```python
from build123d import *

# Parameters (mm, degrees)
SKETCH_1_W          = 855
SKETCH_1_H          = 1200
SKETCH_1_W_2        = 695
SKETCH_1_H_2        = 1040
EXTRUDE_1_DEPTH     = 200
SKETCH_2_W          = 715
SKETCH_2_H          = 1060
CUT_EXTRUDE_1_DEPTH = 10


with BuildPart() as part:
    # Эскиз1 → Вытянуть-Тонкостенный1 (new body)
    with BuildSketch(Plane(origin=(0, 0, 0), x_dir=(1, 0, 0), z_dir=(0, 1, 0))):
        Rectangle(SKETCH_1_W, SKETCH_1_H)
        Rectangle(SKETCH_1_W_2, SKETCH_1_H_2, mode=Mode.SUBTRACT)
    extrude(amount=EXTRUDE_1_DEPTH)

    # Эскиз2 → Вырез-Вытянуть1 (cut)
    with BuildSketch(Plane(origin=(0, 200, 0), x_dir=(1, 0, 0), z_dir=(0, 1, 0))):
        Rectangle(SKETCH_2_W, SKETCH_2_H)
    extrude(amount=-CUT_EXTRUDE_1_DEPTH, mode=Mode.SUBTRACT)


solid = part.part
```
Geometry: final body of the model. Coordinates: model frame, mm. A direction names the side the tool comes from. Round coordinates to 2 decimals unless told otherwise and drop trailing zeros. Order: outer loops, then holes, each group sorted by start corner. A loop starts at its lowest first (then second) coordinate and runs counter-clockwise, first axis right, second up. Notation, with made-up numbers: M 89,-27 L 107,-27 A27 cw 107,-7 Z; hole C 51,-13.5 d11. An arc over 180 degrees is marked long. Use one line per item in the form item = value. Start each with the question number.
Q1. Access query for faces 5 (the face through (-5, 94, 520)), 6 (the face through (-427.5, 99, 8)). Directions: +Z, -Z, +X, -X, +Y, -Y. A direction counts if a zero-diameter tool reaches every point of the face in a straight line with its end or side. Return the directions, or none.
Q2. Mould query, pull axis X, two halves, no side actions, for faces 1 (the face through (374, 0, -8)), 2 (the face through (347.5, 94, 7)), 3 (the face through (-347.5, 94, 7)), 4 (the face through (427.5, 99, 8)). Classes: +X half, -X half, draft (parallel to the pull), parting line (faces both ways), or undercut.
Q3. Cut plane A-A (x = 27). Return loops of the section in (y, z).
Q4. Material intervals for line 1 (Z direction, x = -215, y = 72.5); line 2 (X direction, y = 60, z = -383); line 3 (Z direction, x = 40, y = 190.5), sorted ascending. Write a range as [from, to].
Q5. Cut plane C-C (y = 47). Return loops of the section in (x, z), and give its area (3 significant figures).
Q6. Cut plane B-B (z = -468). Return loops of the section in (x, y), and give its area (3 significant figures).
Geometry results:
q1.face_5 = +Y, -Y
q1.face_6 = +Z, -Z, -X, +Y, -Y
q2.face_1 = draft
q2.face_2 = undercut
q2.face_3 = undercut
q2.face_4 = +X half
q3.outline = M 0,-600 L 200,-600 L 200,-530 L 190,-530 L 190,-520 L 0,-520 Z; M 0,520 L 190,520 L 190,530 L 200,530 L 200,600 L 0,600 Z
q4.line_1 = [-600, -520], [520, 600]
q4.line_2 = [-427.5, -347.5], [347.5, 427.5]
q4.line_3 = [-600, -530], [530, 600]
q5.outline = M -427.5,-600 L 427.5,-600 L 427.5,600 L -427.5,600 Z; hole M -347.5,-520 L 347.5,-520 L 347.5,520 L -347.5,520 Z
q5.area = 303,000 mm^2
q6.outline = M -427.5,0 L -347.5,0 L -347.5,190 L -357.5,190 L -357.5,200 L -427.5,200 Z; M 347.5,0 L 427.5,0 L 427.5,200 L 357.5,200 L 357.5,190 L 347.5,190 Z
q6.area = 31,800 mm^2
